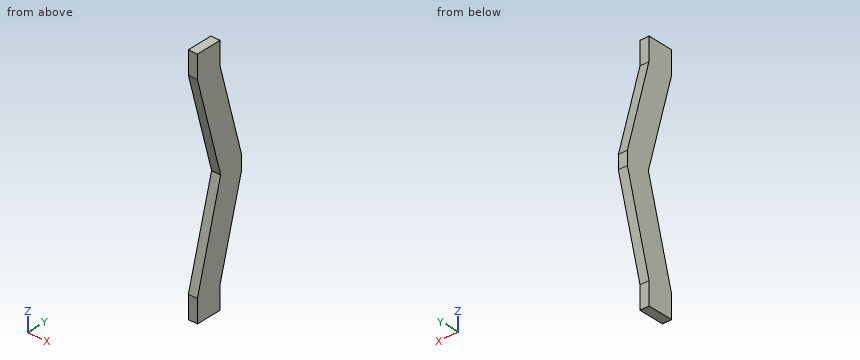
from build123d import *

# Parameters (mm, degrees)
BOSS_EXTRUDE1_DEPTH = 10


with BuildPart() as part:
    # Sketch1 → Boss-Extrude1 (new body)
    with BuildSketch(Plane(origin=(0, 0, 0), x_dir=(0, 0, -1), z_dir=(1, 0, 0))):
        Polygon((0, 0), (-25, 0), (-132.5, 28.804538186), (-240, 0), (-265, 0), (-265, 28), (-240, 28), (-140, 54.794919243), (-125, 54.794919243), (-25, 28), (0, 28), align=None)
    extrude(amount=BOSS_EXTRUDE1_DEPTH)


solid = part.part
Can you work these out from the model? Positions are in its coordinate system, mm. Give positions to 0.01 mm unless a question says otherwise; leave off trailing zeros. Order: outer loops, then holes, each group sorted by start corner. A loop starts at its lowest first (then second) coordinate and runs counter-clockwise, first axis right, second up. Notation, with made-up numbers: M 63,62 L 68,62 A20 cw 68,91 Z; hole C -14,-30.5 d10. An arc over 180 degrees is marked long. One line per question, with ' | ' between items.
Item 1: Please list where these lines run through material, in increasing order: L1, parallel to Y at x = 7.5, z = 20.5; L2, parallel to Y at x = 2.25, z = 231.
Answer block:
L1: y = 0 to 28 | L2: y = 2.41 to 30.41
Item 2: I'm going to push flat-ended pins straight in: pin 1 Ø2 at (x, y) = (1.5, 14.5) entering from -Z; pin 2 Ø5 at (x, z) = (8.5, 86) entering from -Y (3 decimals); pin 3 Ø5 at (x, z) = (6, 13) entering from +Y; pin 4 Ø4 at (x, z) = (1.5, 162.5) entering from -Y. Where does each tip first touch, or does it pass through?
Answer block:
pin 1: stops at z = 0 | pin 2: stops at y = 15.675 | pin 3: stops at y = 28 | pin 4: stops at y = 20.23
Item 3: Suppose I cut it at A-A, the plane y = 16.5. Write out the boundary of the cut face in (x, z).
Answer block:
outline: M 0,0 L 10,0 L 10,86.58 L 0,86.58 Z; M 0,178.42 L 10,178.42 L 10,265 L 0,265 Z
Item 4: Suppose I cut it at C-C, the plane y = 34. Write out the boundary of the cut face in (x, z).
Answer block:
outline: M 0,47.39 L 10,47.39 L 10,217.61 L 0,217.61 Z
Item 5: Suppose I cut it at B-B, the plane x = 8.25. Write out the boundary of the cut face in (y, z), then the cut area to 3 significant figures.
Answer block:
outline: M 0,0 L 28,0 L 28,25 L 54.79,125 L 54.79,140 L 28,240 L 28,265 L 0,265 L 0,240 L 28.8,132.5 L 0,25 Z | area: 7,400 mm2
Item 6: Suppose I cut it at D-D, the plane z = 130. Write out the boundary of the cut face in (x, y), then the cut area to 3 significant figures.
Answer block:
outline: M 0,28.13 L 10,28.13 L 10,54.79 L 0,54.79 Z | area: 267 mm2
